Build history of the part. All positions in model axes, mm. A direction names the side the tool comes from. Give positions to 0.01 mm unless a question says otherwise; leave off trailing zeros. Order: outer loops, then holes, each group sorted by start corner. A loop starts at its lowest first (then second) coordinate and runs counter-clockwise, first axis right, second up. Notation, with made-up numbers: M 42,-29 L 78,-29 A29 cw 78,-4 Z; hole C 76,61 d2. An arc over 180 degrees is marked long. Use CSV: the item, a comma, the result in double quotes. Start each with the question number.
Item 1: Band-saw the part on A-A on y = 54. Write the cut outline in (x, z).
Item 2: Band-saw the part on B-B on x = 25. Write the cut outline in (y, z), plus the area to 3 significant figures.
Item 3: Which spindle directions (+Z, -Z, +X, -X, +Y, -Y) get a long thin tool onto all of the face, cutting with end or side? Do faces 1 (the flat face through (24.65, 4.93, 2.927)), 2 (the cylindrical face through (24.8, 160.5, 12.7)). Say none if no direction does.
Item 4: Wall check: line 1 along X through (y, z) = (99, 11.5); line 2 along Y through (x, z) = (30, 13); line 3 along Y through (x, z) = (26, 3.75). Give the ranges that are in metal, low to high.
Item 5: Two-plate mould, pull along X, no slides. Class faces 3 (the flat face through (14.5, 99, 13)), 4 (the flat face through (50, 86, 12)), 5 (the flat face through (36, 89, 25)): pulls with the +X half, pulls with the -X half, needs draft (parallel to the pull), parting line crosses it, or undercut.
Item 6: Band-saw the part on D-D on z = 4.25. Write the cut outline in (x, y).
Item 7: Band-saw the part on C-C on z = 15.25. Write the cut outline in (x, y).
from build123d import *

# Parameters (mm, degrees)
SKETCH_1_W          = 50
SKETCH_1_H          = 175
EXTRUDE_1_DEPTH     = 25
CUT_EXTRUDE_1_DEPTH = 26
CHAMFER_1_SIZE      = 10
CHAMFER_1_SIZE2     = 5.773502692


with BuildPart() as part:
    # Эскиз1 → Бобышка-Вытянуть1 (new body)
    with BuildSketch(Plane.XY):
        with Locations((25, 87.5)):
            Rectangle(SKETCH_1_W, SKETCH_1_H)
    extrude(amount=EXTRUDE_1_DEPTH)

    # Эскиз2 → Вырез-Вытянуть1 (cut, through all)
    with BuildSketch(Plane.XY.offset(25)):
        with BuildLine():
            Line((14.5, 50), (14.5, 150))
            ThreePointArc((14.5, 150), (25, 160.5), (35.5, 150))
            Line((35.5, 150), (35.5, 50))
            ThreePointArc((35.5, 50), (25, 39.5), (14.5, 50))
        make_face()
    extrude(amount=-CUT_EXTRUDE_1_DEPTH, mode=Mode.SUBTRACT)

    # Фаска1
    chamfer_1_edges = [part.edges().sort_by_distance(p)[0] for p in [
        (25, 0, 0),
    ]]
    chamfer_1_side = [part.faces().sort_by_distance(p)[0] for p in [
        (25, 1.820027472, 0),
    ]]
    chamfer(chamfer_1_edges, length=CHAMFER_1_SIZE, length2=CHAMFER_1_SIZE2, reference=chamfer_1_side[0])


solid = part.part
Model answer:
1,outline,"M 0,0 L 14.5,0 L 14.5,25 L 0,25 Z; M 35.5,0 L 50,0 L 50,25 L 35.5,25 Z"
2,outline,"M 0,5.77 L 10,0 L 39.5,0 L 39.5,25 L 0,25 Z; M 160.5,0 L 175,0 L 175,25 L 160.5,25 Z"
2,area,"1,320 mm^2"
3,face 1,"-Z, +X, -X, -Y"
3,face 2,"+Z, -Z"
4,line 1,"x = 0 to 14.5, 35.5 to 50"
4,line 2,"y = 0 to 40.77, 159.23 to 175"
4,line 3,"y = 3.5 to 39.55, 160.45 to 175"
5,face 3,"undercut"
5,face 4,"pulls with the +X half"
5,face 5,"needs draft"
6,outline,"M 0,2.64 L 50,2.64 L 50,175 L 0,175 Z; hole M 14.5,50 A10.5 ccw 35.5,50 L 35.5,150 A10.5 ccw 14.5,150 Z"
7,outline,"M 0,0 L 50,0 L 50,175 L 0,175 Z; hole M 14.5,50 A10.5 ccw 35.5,50 L 35.5,150 A10.5 ccw 14.5,150 Z"
